Design review of the part shown in the three views and the two pictorial views. Dimensions are in mm from the part's minimum x, y and z. Round coordinates to 2 decimals unless told otherwise and drop trailing zeros. Order: outer loops, then holes, each group sorted by start corner. A loop starts at its lowest first (then second) coordinate and runs counter-clockwise, first axis right, second up.
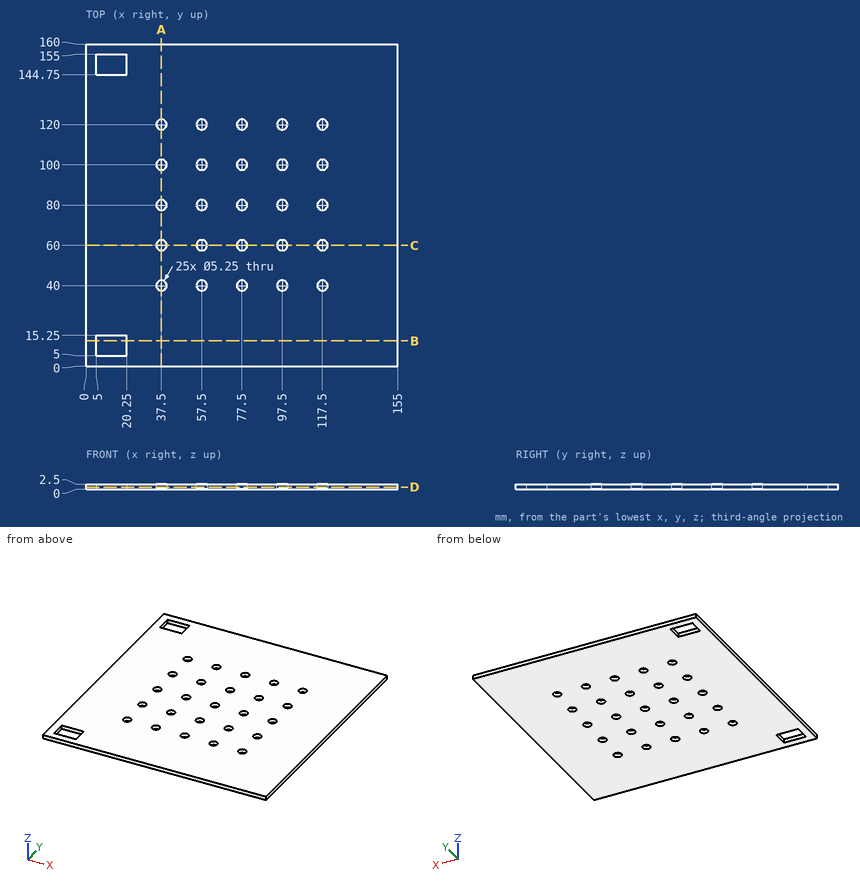
(1) To check wall thickness, follow probe 1 along Y at (x, z) = (77.5, 1.7) (3 decimals); probe 2 along X at (y, z) = (78.5, 0.5); probe 3 along Y at (x, z) = (14, 1.65). State the ranges of each line that lie inside material, in increasing order.
Data:
probe 1: y = 0 to 37.375, 42.625 to 57.375, 62.625 to 77.375, 82.625 to 97.375, 102.625 to 117.375, 122.625 to 160
probe 2: x = 0 to 35.35, 39.65 to 55.35, 59.65 to 75.35, 79.65 to 95.35, 99.65 to 115.35, 119.65 to 155
probe 3: y = 0 to 5, 15.25 to 144.75, 155 to 160
(2) Consider section B-B (y = 12.5). Write out the cut boundary in (x, z), and give its area (3 significant figures).
Data:
outline: (0, 0) - (5, 0) - (5, 2.5) - (0, 2.5) - close; (20.25, 0) - (155, 0) - (155, 2.5) - (20.25, 2.5) - close
area: 349 mm2
(3) Consider section C-C (y = 60). Write out the cut boundary in (x, z) (3 decimals).
Data:
outline: (0, 0) - (34.875, 0) - (34.875, 2.5) - (0, 2.5) - close; (40.125, 0) - (54.875, 0) - (54.875, 2.5) - (40.125, 2.5) - close; (60.125, 0) - (74.875, 0) - (74.875, 2.5) - (60.125, 2.5) - close; (80.125, 0) - (94.875, 0) - (94.875, 2.5) - (80.125, 2.5) - close; (100.125, 0) - (114.875, 0) - (114.875, 2.5) - (100.125, 2.5) - close; (120.125, 0) - (155, 0) - (155, 2.5) - (120.125, 2.5) - close
(4) Consider section D-D (z = 0.9). State how many separate pieces and enclosed holes the cut face has, and give its area (3 significant figures).
Data:
separate pieces: 1
enclosed holes: 27
area: 23,900 mm2
(5) Consider section A-A (x = 37.5). Write out the cut boundary in (y, z) (3 decimals).
Data:
outline: (0, 0) - (37.375, 0) - (37.375, 2.5) - (0, 2.5) - close; (42.625, 0) - (57.375, 0) - (57.375, 2.5) - (42.625, 2.5) - close; (62.625, 0) - (77.375, 0) - (77.375, 2.5) - (62.625, 2.5) - close; (82.625, 0) - (97.375, 0) - (97.375, 2.5) - (82.625, 2.5) - close; (102.625, 0) - (117.375, 0) - (117.375, 2.5) - (102.625, 2.5) - close; (122.625, 0) - (160, 0) - (160, 2.5) - (122.625, 2.5) - close
